from build123d import *

# Parameters (mm, degrees)
SKETCH_1_W          = 5
SKETCH_1_H          = 60
SKETCH_1_W_2        = 30
SKETCH_1_H_2        = 5
SKETCH_1_W_3        = 15
EXTRUDE_1_DEPTH     = 5
FILLET_1_R          = 5
SKETCH_2_W          = 245
SKETCH_2_H          = 125
CUT_EXTRUDE_1_DEPTH = 5
SKETCH_3_W          = 110
SKETCH_3_H          = 2.5
SKETCH_3_W_2        = 115
CUT_EXTRUDE_2_DEPTH = 10
SKETCH_4_W          = 5
SKETCH_4_H          = 5
CUT_EXTRUDE_3_DEPTH = 5
SKETCH_5_W          = 50
SKETCH_5_H          = 44
EXTRUDE_2_DEPTH     = 47
SKETCH_6_W          = 41.4
SKETCH_6_H          = 41.4
CUT_EXTRUDE_4_DEPTH = 47
SKETCH_7_R          = 10.5
CUT_EXTRUDE_5_DEPTH = 316.582224557
CUT_EXTRUDE_6_DEPTH = 44
SKETCH_10_R         = 2
CUT_EXTRUDE_7_DEPTH = 316.582224557
SKETCH_13_R         = 25
CUT_EXTRUDE_9_DEPTH = 20
FILLET_11_R         = 1.497


with BuildPart() as part:
    # 草圖1 → 填料-伸長1 (new body)
    with BuildSketch(Plane(origin=(0, 0, 0), x_dir=(1, 0, 0), z_dir=(0, 1, 0))):
        Polygon((198.746286718, -286.464902661), (198.746286718, -256.464902661), (183.246286718, -256.464902661), (183.246286718, -266.464902661), (124.746286718, -266.464902661), (124.746286718, -262.464902661), (109.246286718, -262.464902661), (109.246286718, -266.464902661), (-21.253713282, -266.464902661), (-21.253713282, 38.535097339), (-36.253713282, 38.535097339), (-36.253713282, 43.535097339), (203.746286718, 43.535097339), (203.746286718, -286.464902661), align=None)
        with Locations((206.246286718, -256.464902661)):
            Rectangle(SKETCH_1_W, SKETCH_1_H)
        with Locations((206.246286718, 13.535097339)):
            Rectangle(SKETCH_1_W, SKETCH_1_H)
        with Locations((188.746286718, 46.035097339)):
            Rectangle(SKETCH_1_W_2, SKETCH_1_H_2)
        with Locations((-21.253713282, 46.035097339)):
            Rectangle(SKETCH_1_W_2, SKETCH_1_H_2)
        with Locations((91.246286718, 46.035097339)):
            Rectangle(SKETCH_1_W_3, SKETCH_1_H_2)
        with Locations((76.246286718, 46.035097339)):
            Rectangle(SKETCH_1_W_3, SKETCH_1_H_2)
        with Locations((206.246286718, -166.464902661)):
            Rectangle(SKETCH_1_W, SKETCH_1_H)
        with Locations((206.246286718, -76.464902661)):
            Rectangle(SKETCH_1_W, SKETCH_1_H)
    extrude(amount=EXTRUDE_1_DEPTH)

    # 圓角1
    fillet_1_edges = [part.edges().sort_by_distance(p)[0] for p in [
        (208.746286718, 5, -13.535097339),
        (208.746286718, 5, 76.464902661),
        (208.746286718, 5, 166.464902661),
        (208.746286718, 5, 256.464902661),
    ]]
    fillet(fillet_1_edges, radius=FILLET_1_R - 0.0001)  # a hair under: the kernel refuses the full size

    # 草圖2 → 除料-伸長1 (cut)
    with BuildSketch(Plane(origin=(0, 5, 0), x_dir=(1, 0, 0), z_dir=(0, 1, 0))):
        with Locations((86.246286718, -13.964902661)):
            Rectangle(SKETCH_2_W, SKETCH_2_H)
    extrude(amount=-CUT_EXTRUDE_1_DEPTH, mode=Mode.SUBTRACT)

    # 草圖3 → 除料-伸長2 (cut)
    with BuildSketch(Plane(origin=(0, 0, 76.464902661), x_dir=(-1, 0, 0), z_dir=(0, 0, -1))):
        with Locations((-33.746286718, 1.25)):
            Rectangle(SKETCH_3_W, SKETCH_3_H)
        with Locations((-151.246286718, 3.75)):
            Rectangle(SKETCH_3_W_2, SKETCH_3_H)
    extrude(amount=-CUT_EXTRUDE_2_DEPTH, mode=Mode.SUBTRACT)

    # 草圖4 → 除料-伸長3 (cut)
    with BuildSketch(Plane(origin=(0, 0, 76.464902661), x_dir=(-1, 0, 0), z_dir=(0, 0, -1))):
        with Locations((-91.246286718, 2.5)):
            Rectangle(SKETCH_4_W, SKETCH_4_H)
    extrude(amount=-CUT_EXTRUDE_3_DEPTH, mode=Mode.SUBTRACT)

    # 草圖5 → 填料-伸長2 (add)
    with BuildSketch(Plane.XY.offset(266.464902661)):
        with Locations((79.746286718, 27)):
            Rectangle(SKETCH_5_W, SKETCH_5_H)
    extrude(amount=-EXTRUDE_2_DEPTH)

    # 草圖6 → 除料-伸長4 (cut)
    with BuildSketch(Plane.ZY.offset(-54.746286718)):
        with Locations((242.964902661, 25.7)):
            Rectangle(SKETCH_6_W, SKETCH_6_H)
    extrude(amount=-CUT_EXTRUDE_4_DEPTH, mode=Mode.SUBTRACT)

    # 草圖7 → 除料-伸長5 (cut, through all)
    with BuildSketch(Plane.ZY.offset(-101.746286718)):
        with Locations((242.964902661, 25.7)):
            Circle(SKETCH_7_R)
    extrude(amount=-CUT_EXTRUDE_5_DEPTH, mode=Mode.SUBTRACT)

    # 草圖8 → 除料-伸長6 (cut)
    with BuildSketch(Plane(origin=(0, 49, 0), x_dir=(1, 0, 0), z_dir=(0, 1, 0))):
        Polygon((54.746286718, -263.664902661), (101.746286718, -222.464902661), (104.746286718, -222.464902661), (104.746286718, -219.464902661), (54.746286718, -219.464902661), align=None)
    extrude(amount=-CUT_EXTRUDE_6_DEPTH, mode=Mode.SUBTRACT)

    # 草圖10 → 除料-伸長7 (cut, through all)
    with BuildSketch(Plane.ZY.offset(-101.746286718)):
        with Locations((227.464902661, 41.4)):
            Circle(SKETCH_10_R)
        with Locations((258.664902661, 41.4)):
            Circle(SKETCH_10_R)
        with Locations((258.664902661, 10)):
            Circle(SKETCH_10_R)
        with Locations((227.464902661, 10)):
            Circle(SKETCH_10_R)
    extrude(amount=-CUT_EXTRUDE_7_DEPTH, mode=Mode.SUBTRACT)

    # 草圖13 → 除料-伸長9 (cut)
    with BuildSketch(Plane(origin=(104.746286718, 0, 0), x_dir=(0, 0, -1), z_dir=(1, 0, 0))):
        with Locations((-242.964902661, 25.7)):
            Circle(SKETCH_13_R)
    extrude(amount=CUT_EXTRUDE_9_DEPTH, mode=Mode.SUBTRACT)

    # 圓角11
    fillet_11_edges = [part.edges().sort_by_distance(p)[0] for p in [
        (54.746286718, 27, 266.464902661),
        (79.746286718, 49, 266.464902661),
        (104.746286718, 27, 266.464902661),
        (104.746286718, 25.7, 232.464902661),
        (54.746286718, 49, 265.064902661),
        (104.746286718, 49, 244.464902661),
        (104.746286718, 27, 222.464902661),
        (78.246286718, 49, 243.064902661),
        (103.246286718, 49, 222.464902661),
    ]]
    fillet(fillet_11_edges, radius=FILLET_11_R)


solid = part.part
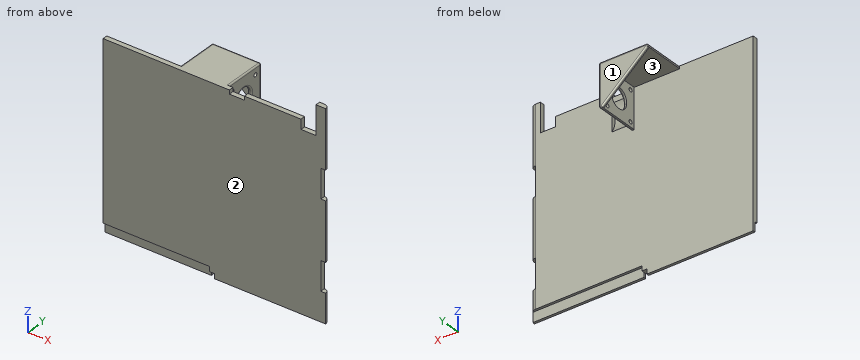
Design review of the part built by this model. Coordinates are the model's own, in mm. Face numbers are marked on the shaded views. Round coordinates to 2 decimals unless told otherwise and drop trailing zeros. Write each loop counter-clockwise with the first axis right and the second up, starting at its lowest first coordinate (ties: lowest second). Pieces come first, ordered by that corner, then holes. Notation, with made-up numbers: (78, -38.5) - (121, -38.5) arc R16 cw to (121, -33.5) - close; hole circle Ø5 at (43, -13.5). An arc over 180 degrees is marked (long way). Use a Markdown table: item, result. Add a question column.
1. Clearance check with flat-ended pins moving along their axes: pin 1 (1.2 mm diameter, centred on y = 3.5, z = 78, fed in from +X); pin 2 (1.2 mm diameter, centred on y = 4, z = 83.5, fed in from +X); pin 3 (2.5 mm diameter, centred on x = 121, y = 2, fed in from +Z). State where each tip first meets the part, or that it passes through.
2. We need section C-C (x = 160.5). State the section outline as (y, z) points, then the cut area to 3 significant figures.
3. Wall thickness on probe 1 along Z at (x, y) = (103, 41); probe 2 along Y at (x, z) = (83.5, 229); probe 3 along Z at (x, y) = (89.5, 17.5): over which ranges is each line inside the solid? List them lowest first.
4. We need section D-D (x = 191). State the section outline as (y, z) points.
5. We need section A-A (y = 25.7). State the section outline as (x, z) points, then the cut area to 3 significant figures.
6. Mouldability with a two-part tool opening along Y and no side actions: class the marked faces 1, 2 and 3 as +Y half, -Y half, draft (parallel to the pull), parting line (faces both ways), or undercut.
Output:
| question | item | result |
|---|---|---|
| 1 | pin 1 | stops at x = 88.75 |
| 1 | pin 2 | stops at x = 93.75 |
| 1 | pin 3 | stops at z = 262.46 |
| 2 | outline | (0, 76.46) - (2.5, 76.46) - (2.5, 86.46) - (5, 86.46) - (5, 266.46) - (0, 266.46) - close |
| 2 | area | 925 mm2 |
| 3 | probe 1 | z = 222.46 to 225.51, 229.42 to 256.71, 260.62 to 266.46 |
| 3 | probe 2 | y = 0 to 5 |
| 3 | probe 3 | z = 263.66 to 266.46 |
| 4 | outline | (0, 76.46) - (2.5, 76.46) - (2.5, 86.46) - (5, 86.46) - (5, 256.46) - (0, 256.46) - close |
| 5 | outline | (54.75, 263.66) - (101.75, 263.66) - (101.75, 253.46) - (103.25, 253.46) arc R1.5 ccw to (104.75, 254.96) - (104.75, 264.97) arc R1.5 ccw to (103.25, 266.46) - (56.24, 266.46) arc R1.5 ccw to (54.75, 264.97) - close; (101.75, 222.46) - (103.25, 222.46) arc R1.5 ccw to (104.75, 223.96) - (104.75, 230.97) arc R1.5 ccw to (103.25, 232.46) - (101.75, 232.46) - close |
| 5 | area | 198 mm2 |
| 6 | face 1 | +Y half |
| 6 | face 2 | -Y half |
| 6 | face 3 | undercut |
